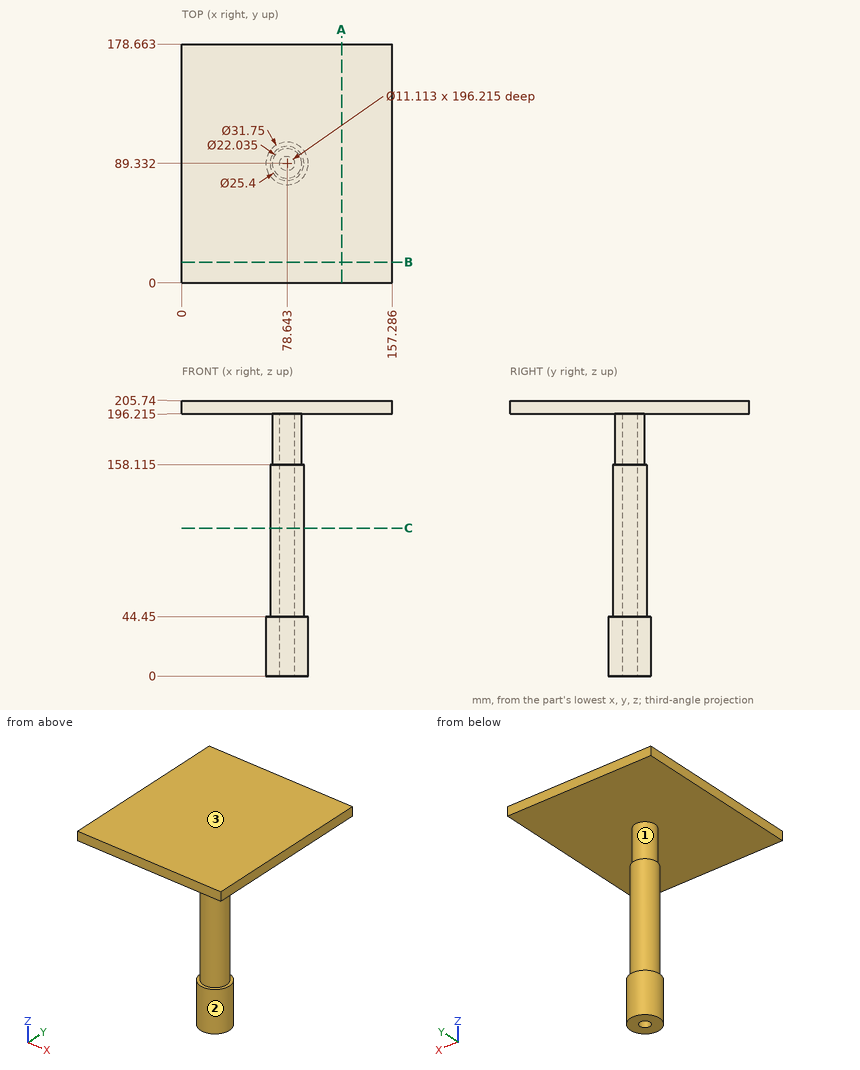
Drawing for the job (mm, zero at the part's lowest x, y, z). A direction names the side the tool comes from. Give positions to 0.01 mm unless a question says otherwise; leave off trailing zeros. Order: outer loops, then holes, each group sorted by start corner. A loop starts at its lowest first (then second) coordinate and runs counter-clockwise, first axis right, second up. Notation, with made-up numbers: M 89.5,5.5 L 138.5,5.5 A26 ccw 138.5,28.5 Z; hole C -25.75,82.25 d8. An arc over 180 degrees is marked long. Use a Markdown table: item, result. Add a question column.
(1) Probe line 1 along Y through (x, z) = (78.5, 127) (1 decimal); line 2 along Z through (x, y) = (11, 162) (1 decimal); line 3 along Y through (x, z) = (79, 188.5). List the from-to ranges inside material, lowest first. Write a range as [from, to].
(2) Drop flat-ended pins along their axis: P1, Ø6, axis at x = 90, z = 115, coming from the +Y side (1 decimal); P2, Ø3.5, axis at x = 76, y = 87, coming from the -Z side (1 decimal). Give the stop position or say it passes through.
(3) Saw through at C-C, the plane z = 110.5. Give the cut face in (x, y), and give its area (3 significant figures).
(4) Saw through at A-A, the plane x = 119.5. Give the cut face in (y, z) (1 decimal), and give its area (3 significant figures).
(5) 3-axis set-ups, long thin cutter, end or side, ignore diameter. For the marked faces 1, 2 and 3: which of +Z, -Z, +X, -X, +Y, -Y reach the whole face in a straight line?
(6) Saw through at B-B, the plane y = 15.5. Give the cut face in (x, z) (1 decimal).
Answer key:
| question | item | result |
|---|---|---|
| 1 | line 1 | [76.6, 83.8], [94.9, 102] |
| 1 | line 2 | [196.2, 205.7] |
| 1 | line 3 | [78.32, 83.79], [94.88, 100.34] |
| 2 | P1 | y = 98.9 |
| 2 | P2 | z = 196.2 |
| 3 | outline | C 78.64,89.33 d25.4; hole C 78.64,89.33 d11.11 |
| 3 | area | 410 mm^2 |
| 4 | outline | M 0,196.2 L 178.7,196.2 L 178.7,205.7 L 0,205.7 Z |
| 4 | area | 1,700 mm^2 |
| 5 | face 1 | none |
| 5 | face 2 | -Z |
| 5 | face 3 | +Z, +X, -X, +Y, -Y |
| 6 | outline | M 0,196.2 L 157.3,196.2 L 157.3,205.7 L 0,205.7 Z |
